```python
from build123d import *

# Parameters (mm, degrees)
BOSS_EXTRUDE1_DEPTH = 20
FILLET1_R           = 3
SKETCH2_R           = 2.5
CUT_EXTRUDE1_DEPTH  = 8
SKETCH3_R           = 2.5
CUT_EXTRUDE2_DEPTH  = 75
SKETCH3_4_R         = 2.5
CUT_EXTRUDE3_DEPTH  = 3.175
FILLET2_R           = 1


with BuildPart() as part:
    # Sketch1 → Boss-Extrude1 (new body)
    with BuildSketch(Plane.XY):
        with BuildLine():
            Line((4, -44.319860108), (4, -63.369860108))
            Line((4, -63.369860108), (9, -63.369860108))
            Line((9, -63.369860108), (9, -48.674942219))
            ThreePointArc((9, -48.674942219), (49.221622989, -5.242311542), (19.05, 45.68749829))
            Line((19.05, 45.68749829), (19.05, 56.55))
            Line((19.05, 56.55), (65, 56.55))
            Line((65, 56.55), (65, 63.55))
            Line((65, 63.55), (-65, 63.55))
            Line((-65, 63.55), (-65, 56.55))
            Line((-65, 56.55), (-19.05, 56.55))
            Line((-19.05, 56.55), (-19.05, 45.68749829))
            ThreePointArc((-19.05, 45.68749829), (-49.221622989, -5.242311542), (-9, -48.674942219))
            Line((-9, -48.674942219), (-9, -63.369860108))
            Line((-9, -63.369860108), (-4, -63.369860108))
            Line((-4, -63.369860108), (-4, -44.319860108))
            ThreePointArc((-4, -44.319860108), (0, 44.5), (4, -44.319860108))
        make_face()
    extrude(amount=BOSS_EXTRUDE1_DEPTH)

    # Fillet1
    fillet1_edges = [part.edges().sort_by_distance(p)[0] for p in [
        (-19.05, 56.55, 10),
        (19.05, 56.55, 10),
        (19.05, 45.68749829, 10),
        (-19.05, 45.68749829, 10),
    ]]
    fillet(fillet1_edges, radius=FILLET1_R)

    # Sketch2 → Cut-Extrude1 (cut, through all)
    with BuildSketch(Plane(origin=(0, 56.55, 0), x_dir=(-1, 0, 0), z_dir=(0, -1, 0))):
        with Locations((55, -10)):
            Circle(SKETCH2_R)
        with Locations((-55, -10)):
            Circle(SKETCH2_R)
    extrude(amount=-CUT_EXTRUDE1_DEPTH, mode=Mode.SUBTRACT)

    # Sketch3 → Cut-Extrude2 (cut, through all)
    with BuildSketch(Plane.ZY.offset(9)):
        with Locations((10, -56.369860108)):
            Circle(SKETCH3_R)
    extrude(amount=-CUT_EXTRUDE2_DEPTH, mode=Mode.SUBTRACT)

    # Sketch3<4> → Cut-Extrude3 (cut)
    with BuildSketch(Plane.ZY.offset(9)):
        Polygon((15.600297611, -56.369860108), (12.800148806, -51.519860108), (7.199851194, -51.519860108), (4.399702389, -56.369860108), (7.199851194, -61.219860108), (12.800148806, -61.219860108), align=None)
        with Locations((10, -56.369860108)):
            Circle(SKETCH3_4_R, mode=Mode.SUBTRACT)
    extrude(amount=-CUT_EXTRUDE3_DEPTH, mode=Mode.SUBTRACT)

    # Fillet2
    fillet2_edges = [part.edges().sort_by_distance(p)[0] for p in [
        (-9, -56.022401163, 20),
        (-6.5, -63.369860108, 20),
        (-4, -53.844860108, 20),
        (0, 44.5, 20),
        (4, -53.844860108, 20),
        (6.5, -63.369860108, 20),
        (9, -56.022401163, 20),
        (49.1118994, -6.186383215, 20),
        (19.05, 50.59750774, 20),
        (43.525, 56.55, 20),
        (-49.1118994, -6.186383215, 20),
        (65, 60.05, 20),
        (-19.05, 50.59750774, 20),
        (19.522155068, 46.029466037, 20),
        (0, 63.55, 20),
        (19.928679656, 55.671320344, 20),
        (-19.522155068, 46.029466037, 20),
        (-19.928679656, 55.671320344, 20),
        (-65, 60.05, 20),
        (-43.525, 56.55, 20),
    ]]
    fillet(fillet2_edges, radius=FILLET2_R)


solid = part.part
```
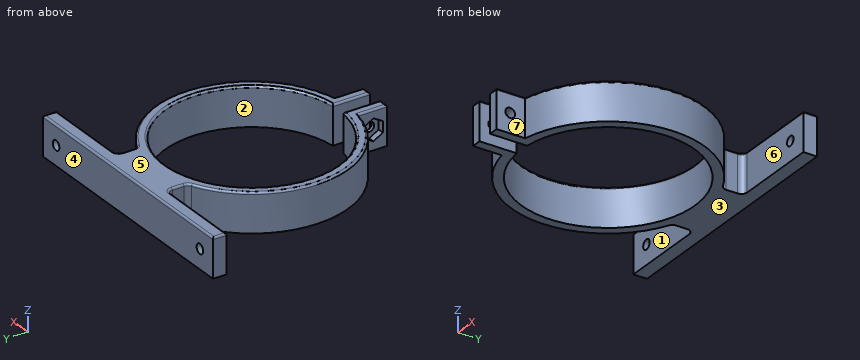
Could you check a few things on this model? Use its own coordinates, in mm. Face numbers are marked on the shaded views. A direction names the side the tool comes from. Coordinates: 2 decimals unless noted, no trailing zeros. Loops run counter-clockwise (first coordinate to the right, second up) from the corner with the lowest first, then second, coordinate; pieces in that order, holes last. Notation, with made-up numbers: M 53,15.5 L 75,15.5 A11 ccw 75,35.5 Z; hole C 61.5,74 d4. An arc over 180 degrees is marked long. Put each result on its own line as item: value. Start each with the question number.
(1) Suppose I cut it at C-C on x = 0. Please give me the cut outline in (y, z).
(2) Thinking about a two-plate mould opening in Y: for the marked faces 1, 2, 3 and 4, which applies, pulls with the +Y half, pulls with the -Y half, needs draft (parallel to the pull), parting line crosses it, or undercut?
(3) Will these pins go through, and if not, where does the flat tip stop? P1, Ø12, axis at x = -32.5, y = -46, coming from the +Z side; P2, Ø6.5, axis at y = -56.37, z = 10, coming from the -X side (3 decimals); P3, Ø2, axis at x = -22.5, z = 12, coming from the -Y side; P4, Ø12, axis at y = -56.5, z = 9.5, coming from the +X side.
(4) I need wall thicknesses on line 1 (X direction, y = 61, z = 10); line 2 (Z direction, x = -55, y = 58.5); line 3 (X direction, y = 0, z = 5.5). Which ranges of each line are inside material? Lowest first, please. Write a range as from..to.
(5) For the marked faces 5, 6 and 7, which set-ups out of +Z, -Z, +X, -X, +Y, -Y let a thin tool reach every point of the face, with its end or its side?
(6) Suppose I cut it at A-A on x = -55. Please give me the cut outline in (y, z).
(7) Suppose I cut it at B-B on z = 10. Count the separate pieces of the cut face and the enclosed holes in it, then the cut area to 3 significant figures.
Solutions:
1. outline: M 44.5,0 L 63.55,0 L 63.55,19 A1 ccw 62.55,20 L 45.5,20 A1 ccw 44.5,19 Z
2. face 1: undercut
2. face 2: undercut
2. face 3: needs draft
2. face 4: pulls with the +Y half
3. P1: passes through
3. P2: stops at x = -5.825
3. P3: stops at y = -44.59
3. P4: stops at x = 9
4. line 1: x = -65..-57.5, -52.5..52.5, 57.5..65
4. line 2: z = 0..7.5, 12.5..20
4. line 3: x = -49.5..-44.5, 44.5..49.5
5. face 5: +Z, +X, -X, +Y, -Y
5. face 6: +Z, -Z, +X
5. face 7: +Z, -Z, +X, -Y
6. outline: M 56.55,0 L 63.55,0 L 63.55,7.5 L 56.55,7.5 Z; M 56.55,12.5 L 63.55,12.5 L 63.55,19 A1 ccw 62.55,20 L 57.55,20 A1 ccw 56.55,19 Z
7. separate pieces: 5
7. enclosed holes: 0
7. area: 2,680 mm2
